from build123d import *

# Parameters (mm, degrees)
F0_W     = 67
F0_H     = 17
F0_R     = 1.5
F1_DEPTH = 3
F2_DEPTH = 14
F3_R     = 5
F4_R     = 0.99999
F5_SIZE  = 2


# Not quite as in the source:
# - a fillet or chamfer is up to 0.001 mm smaller than in the source, because OpenCascade refuses the exact size


with BuildPart() as f1:
    # F0 (on Front) → F1 (new body)
    with BuildSketch(Plane.XZ):
        Polygon((-33.5, 18.5), (-33.5, 8.5), (33.5, 8.5), (33.5, 18.5), (1, 18.5), (1, 11), (-1, 11), (-1, 18.5), align=None)
        Rectangle(F0_W, F0_H)
        with Locations((-25, 0)):
            Circle(F0_R, mode=Mode.SUBTRACT)
        with Locations((25, 0)):
            Circle(F0_R, mode=Mode.SUBTRACT)
    extrude(amount=F1_DEPTH)

    # F0 (on Front) → F2 (join)
    with BuildSketch(Plane.XZ):
        Polygon((-33.5, 22.5), (-33.5, 18.5), (-1, 18.5), (-1, 19), (1, 19), (1, 18.5), (33.5, 18.5), (33.5, 22.5), align=None)
    extrude(amount=F2_DEPTH)

    # F3
    f3_edges = [f1.edges().sort_by_distance(p)[0] for p in [
        (-33.5, -1.5, -8.5),
        (33.5, -1.5, -8.5),
        (-33.5, -7, 22.5),
        (33.5, -7, 22.5),
    ]]
    fillet(f3_edges, radius=F3_R)

    # F4 (radius 1 in the source; OpenCascade refuses exactly that, so slightly less here)
    f4_edges = [f1.edges().sort_by_distance(p)[0] for p in [
        (-1, -7, 19),
        (1, -7, 19),
        (1, -1.5, 11),
        (-1, -1.5, 11),
    ]]
    fillet(f4_edges, radius=F4_R)

    # F5
    f5_edges = [f1.edges().sort_by_distance(p)[0] for p in [
        (-26.5, 0, 0),
        (23.5, 0, 0),
        (-1, 0, 15),
    ]]
    chamfer(f5_edges, length=F5_SIZE)


solid = f1.part
Check sheet for the modelled part. Datum: model origin and axes. Units: mm. A direction names the side the tool comes from. Give positions to 0.01 mm unless a question says otherwise; leave off trailing zeros. Write each loop counter-clockwise with the first axis right and the second up, starting at its lowest first coordinate (ties: lowest second). Pieces come first, ordered by that corner, then holes. Notation, with made-up numbers: M -34.5,17.25 L -17.5,17.25 A22 cw -17.5,40.25 Z; hole C -34,74.5 d6. An arc over 180 degrees is marked long. Use one line per item in the form item = value.
(1) Section check B-B on x = 25. Record the boundary of the cut face in (y, z), plus the area to 3 significant figures.
Answer block:
outline = M -14,18.5 L -3,18.5 L -3,1.5 L -2,1.5 L 0,3.5 L 0,22.5 L -14,22.5 Z; M -3,-8.5 L 0,-8.5 L 0,-3.5 L -2,-1.5 L -3,-1.5 Z
area = 124 mm2
(2) Material ranges on line 1 along Z through (x, y) = (25, -2.7); line 2 along Y through (x, z) = (3.5, -6.5); line 3 along Z through (x, y) = (-16, -8), recorded low to high.
Answer block:
line_1 = -8.5 to -1.5, 1.5 to 22.5
line_2 = -3 to 0
line_3 = 18.5 to 22.5
(3) Tool access check on faces 1 (the flat face through (-33.5, -1, 7)), 2 (the flat face through (17, -8, 18.5)), 3 (the conical face through (-1.44, -0.986, 10.592)). Record the directions out of +Z, -Z, +X, -X, +Y, -Y that give a thin tool (end or side, any length) a straight path to the whole face; none if there is none.
Answer block:
face_1 = +Z, -Z, -X, +Y, -Y
face_2 = -Z, +X, -X, -Y
face_3 = +Y
(4) Draft check along Z on faces 4 (the flat face through (-2, -1, 15)), 5 (the flat face through (-17, -8, 18.5)), 6 (the flat face through (0, -7, 22.5)). Enter one of: pulls with the +Z half, pulls with the -Z half, needs draft (parallel to the pull), parting line crosses it, or undercut.
Answer block:
face_4 = undercut
face_5 = pulls with the -Z half
face_6 = pulls with the +Z half
(5) Section check A-A on z = 0. Record the boundary of the cut face in (x, y), plus the area to 3 significant figures.
Answer block:
outline = M -33.5,-3 L -26.5,-3 L -26.5,-2 L -28.5,0 L -33.5,0 Z; M -23.5,-3 L 23.5,-3 L 23.5,-2 L 21.5,0 L -21.5,0 L -23.5,-2 Z; M 26.5,-3 L 33.5,-3 L 33.5,0 L 28.5,0 L 26.5,-2 Z
area = 175 mm2
(6) Section check D-D on x = 11.5. Record the boundary of the cut face in (y, z), plus the area to 3 significant figures.
Answer block:
outline = M -14,18.5 L -3,18.5 L -3,-8.5 L 0,-8.5 L 0,22.5 L -14,22.5 Z
area = 137 mm2
(7) Depth check by flat-ended pin: P1, Ø2.5, axis at x = 25, z = 0, coming from the +Y side; P2, Ø3.5, axis at x = 20.5, y = -7.5, coming from the -Z side; P3, Ø8, axis at x = 9, z = -4, coming from the -Y side; P4, Ø5, axis at y = -8, z = 19, coming from the -X side. Enter the tip coordinate at first touch or a pass-through.
Answer block:
P1 = through
P2 = 18.5
P3 = -3
P4 = -33.4
